Design review of the part built by this model. Coordinates are the model's own, in mm. Give positions to 0.01 mm unless a question says otherwise; leave off trailing zeros. Loops run counter-clockwise (first coordinate to the right, second up) from the corner with the lowest first, then second, coordinate; pieces in that order, holes last. Notation, with made-up numbers: (77.25, -12) -> (94.25, -12) arc R20 cw to (94.25, -5) -> close; hole circle Ø7 at (65, 17). An arc over 180 degrees is marked (long way). Answer as CSV lines item,"result".
from build123d import *

# Parameters (mm, degrees)
ESQUISSE1_W             = 203.2
ESQUISSE1_H             = 203.2
BOSS_EXTRU_1_DEPTH      = 6.35
ESQUISSE2_R             = 2.5
ENL_V_MAT_EXTRU_1_DEPTH = 144.824345992
ESQUISSE3_R             = 2.5
ENL_V_MAT_EXTRU_2_DEPTH = 144.824345992
ESQUISSE4_R             = 2.5
ENL_V_MAT_EXTRU_3_DEPTH = 144.824345992


with BuildPart() as part:
    # Esquisse1 → Boss.-Extru.1 (new body)
    with BuildSketch(Plane(origin=(0, 0, 0), x_dir=(1, 0, 0), z_dir=(0, 1, 0))):
        Rectangle(ESQUISSE1_W, ESQUISSE1_H)
    extrude(amount=BOSS_EXTRU_1_DEPTH)

    # Esquisse2 → Enlèv. mat.-Extru.1 (cut, through all)
    with BuildSketch(Plane(origin=(0, 6.35, 0), x_dir=(1, 0, 0), z_dir=(0, 1, 0))):
        with Locations(Location((-33.725, -49.85, 0), (0, 0, 270))):
            Circle(ESQUISSE2_R)
        with Locations(Location((-33.725, -79.85, 0), (0, 0, 270))):
            Circle(ESQUISSE2_R)
        with Locations(Location((33.425, -79.85, 0), (0, 0, 270))):
            Circle(ESQUISSE2_R)
        with Locations(Location((33.425, -49.85, 0), (0, 0, 270))):
            Circle(ESQUISSE2_R)
    extrude(amount=-ENL_V_MAT_EXTRU_1_DEPTH, mode=Mode.SUBTRACT)

    # Esquisse3 → Enlèv. mat.-Extru.2 (cut, through all)
    with BuildSketch(Plane(origin=(0, 6.35, 0), x_dir=(1, 0, 0), z_dir=(0, 1, 0))):
        with Locations(Location((-93.6, 93.6, 0), (0, 0, 270))):
            Circle(ESQUISSE3_R)
        with Locations(Location((93.6, 93.6, 0), (0, 0, 270))):
            Circle(ESQUISSE3_R)
        with Locations(Location((93.6, -93.6, 0), (0, 0, 270))):
            Circle(ESQUISSE3_R)
        with Locations(Location((-93.6, -93.6, 0), (0, 0, 270))):
            Circle(ESQUISSE3_R)
    extrude(amount=-ENL_V_MAT_EXTRU_2_DEPTH, mode=Mode.SUBTRACT)

    # Esquisse4 → Enlèv. mat.-Extru.3 (cut, through all)
    with BuildSketch(Plane(origin=(0, 6.35, 0), x_dir=(1, 0, 0), z_dir=(0, 1, 0))):
        with Locations(Location((-15.588457268, 74, 0), (0, 0, 270))):
            Circle(ESQUISSE4_R)
        with Locations(Location((15.588457268, 74, 0), (0, 0, 270))):
            Circle(ESQUISSE4_R)
        with Locations(Location((0, 47, 0), (0, 0, 270))):
            Circle(ESQUISSE4_R)
        with Locations(Location((-75, -83, 0), (0, 0, 270))):
            Circle(ESQUISSE4_R)
        with Locations(Location((-90.588457268, -56, 0), (0, 0, 270))):
            Circle(ESQUISSE4_R)
        with Locations(Location((-59.411542732, -56, 0), (0, 0, 270))):
            Circle(ESQUISSE4_R)
        with Locations(Location((59.411542732, -56, 0), (0, 0, 270))):
            Circle(ESQUISSE4_R)
        with Locations(Location((90.588457268, -56, 0), (0, 0, 270))):
            Circle(ESQUISSE4_R)
        with Locations(Location((75, -83, 0), (0, 0, 270))):
            Circle(ESQUISSE4_R)
    extrude(amount=-ENL_V_MAT_EXTRU_3_DEPTH, mode=Mode.SUBTRACT)


solid = part.part
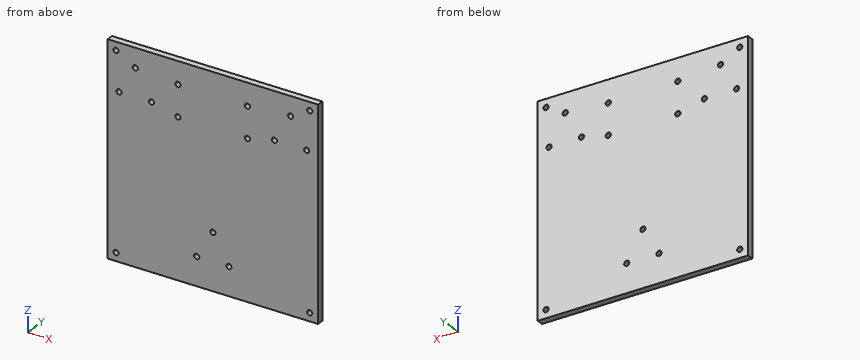
Q1. We need section A-A, the plane x = -75. State the section outline as (y, z) points.
Filled sheet:
outline,"(0, -101.6) -> (6.35, -101.6) -> (6.35, 80.5) -> (0, 80.5) -> close; (0, 85.5) -> (6.35, 85.5) -> (6.35, 101.6) -> (0, 101.6) -> close"
Q2. We need section B-B, the plane z = -74. State the section outline as (x, y) points.
Filled sheet:
outline,"(-101.6, 0) -> (-18.09, 0) -> (-18.09, 6.35) -> (-101.6, 6.35) -> close; (-13.09, 0) -> (13.09, 0) -> (13.09, 6.35) -> (-13.09, 6.35) -> close; (18.09, 0) -> (101.6, 0) -> (101.6, 6.35) -> (18.09, 6.35) -> close"
Q3. To check wall thickness, follow probe 1 along X at (y, z) = (2.75, -47); probe 2 along X at (y, z) = (4.25, 49.85) (3 decimals); probe 3 along X at (y, z) = (4.5, 56). State the ranges of each line that lie inside material, in increasing order. Write a range as from..to.
Filled sheet:
probe 1,"x = -101.6..-2.5, 2.5..101.6"
probe 2,"x = -101.6..-36.225, -31.225..30.925, 35.925..101.6"
probe 3,"x = -101.6..-93.09, -88.09..-61.91, -56.91..56.91, 61.91..88.09, 93.09..101.6"
Q4. Clearance check with a flat-ended pin moving along its axis: pin 1 Ø10 at (x, z) = (43, -40) entering from -Y. State where the tip first meets the part, or that it passes through.
Filled sheet:
pin 1,"stops at y = 0"
